Model file for the job. Use its own axes, mm. Face numbers are marked on the shaded views. A direction names the side the tool comes from. Round coordinates to 2 decimals unless told otherwise and drop trailing zeros. Order: outer loops, then holes, each group sorted by start corner. A loop starts at its lowest first (then second) coordinate and runs counter-clockwise, first axis right, second up. Notation, with made-up numbers: M 15,52.25 L 40,52.25 A13 ccw 40,56.25 Z; hole C 89,49.5 d4. An arc over 180 degrees is marked long. Return JSON: item names as keys, results as strings. Group by question number.
Item 1: Slice it at B-B on y = 4.25. Write the cut outline in (x, z).
Item 2: Slice it at A-A on z = -27. Write the cut outline in (x, y).
Item 3: Probe line 1 along X through (y, z) = (4.05, -29.5); line 2 along Z through (x, y) = (80.5, 3.55); line 3 along Z through (x, y) = (16.5, 3.7). List the from-to ranges inside material, lowest first.
Item 4: Pull direction Z, two halves, no side cores. Call the marked faces 3 and 4: pulls with the +Z half, pulls with the -Z half, needs draft (parallel to the pull), parting line crosses it, or undercut.
Item 5: Slice it at D-D on x = 66. Write the cut outline in (y, z).
Item 6: Slice it at C-C on x = -88. Write the cut outline in (y, z).
Item 7: Pin check, flat tips, straight feed: pin 1 Ø16 at (x, z) = (15, 89) entering from +Y; pin 2 Ø2 at (y, z) = (4, 86) entering from +X; pin 3 Ø3 at (x, y) = (-47, 3) entering from +Z. Stop position of each tip, or through.
Item 8: Which spindle directions (+Z, -Z, +X, -X, +Y, -Y) get a long thin tool onto all of the face, cutting with end or side? Do the marked faces 1 and 2. Say none if no direction does.
from build123d import *

# Parameters (mm, degrees)
BOSS_EXTRUDE1_DEPTH = 5
CUT_EXTRUDE4_START  = 5
SKETCH1_5_R         = 10
CUT_EXTRUDE4_DEPTH  = 1.6
CIRPATTERN1_COUNT   = 3


with BuildPart() as part:
    # Sketch1 → Boss-Extrude1 (new body)
    with BuildSketch(Plane(origin=(0, 0, 0), x_dir=(1, 0, 0), z_dir=(0, 1, 0))):
        Polygon((20, -105.358983849), (101.24355653, 35.358983849), (81.24355653, 70), (-81.24355653, 70), (-101.24355653, 35.358983849), (-20, -105.358983849), align=None)
    extrude(amount=BOSS_EXTRUDE1_DEPTH)

    # Sketch1<5> → Cut-Extrude4 (cut)
    with BuildSketch(Plane(origin=(0, 0, 0), x_dir=(1, 0, 0), z_dir=(0, 1, 0)).offset(CUT_EXTRUDE4_START)):
        with Locations(Location((-14.186994533, -87.858983849, 0), (0, 0, 270))):
            Circle(SKETCH1_5_R)
        with Locations(Location((14.186994533, -87.858983849, 0), (0, 0, 270))):
            Circle(SKETCH1_5_R)
    cut_extrude4 = extrude(amount=-CUT_EXTRUDE4_DEPTH, mode=Mode.SUBTRACT)

    # CirPattern1: Cut-Extrude4 ×3 about axis
    cirpattern1_axis = Axis((0, 0, 0), (0, 1, 0))
    for i in range(1, CIRPATTERN1_COUNT):
        add(cut_extrude4.rotate(cirpattern1_axis, i * 360 / CIRPATTERN1_COUNT), mode=Mode.SUBTRACT)


solid = part.part
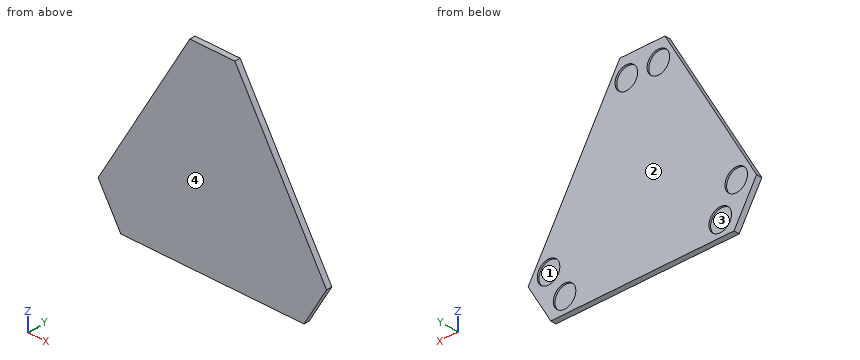
Output values:
{
 "1": {"outline": "M -101.24,-35.36 L -81.24,-70 L 81.24,-70 L 101.24,-35.36 L 20,105.36 L -20,105.36 Z; hole C -83.18,-31.64 d20; hole C -68.99,-56.22 d20; hole C -14.19,87.86 d20; hole C 14.19,87.86 d20; hole C 68.99,-56.22 d20; hole C 83.18,-31.64 d20"},
 "2": {"outline": "M -96.42,0 L 96.42,0 L 96.42,5 L 92.04,5 L 92.04,3.4 L 74.32,3.4 L 74.32,5 L -74.32,5 L -74.32,3.4 L -92.04,3.4 L -92.04,5 L -96.42,5 Z"},
 "3": {"line 1": "-97.86 to -92.95, -73.41 to 73.41, 92.95 to 97.86", "line 2": "-70 to -41.28, -22.01 to 0.57", "line 3": "-70 to 78.13, 97.59 to 105.36"},
 "4": {"face 3": "undercut", "face 4": "needs draft"},
 "5": {"outline": "M 0,-70 L 5,-70 L 5,-65.76 L 3.4,-65.76 L 3.4,-46.67 L 5,-46.67 L 5,25.68 L 0,25.68 Z"},
 "6": {"outline": "M 0,-58.3 L 5,-58.3 L 5,-40.41 L 3.4,-40.41 L 3.4,-22.88 L 5,-22.88 L 5,-12.42 L 0,-12.42 Z"},
 "7": {"pin 1": "y = 3.4", "pin 2": "x = 31.75", "pin 3": "z = 61.19"},
 "8": {"face 1": "+Y", "face 2": "+Z, -Z, +X, -X, +Y"}
}
